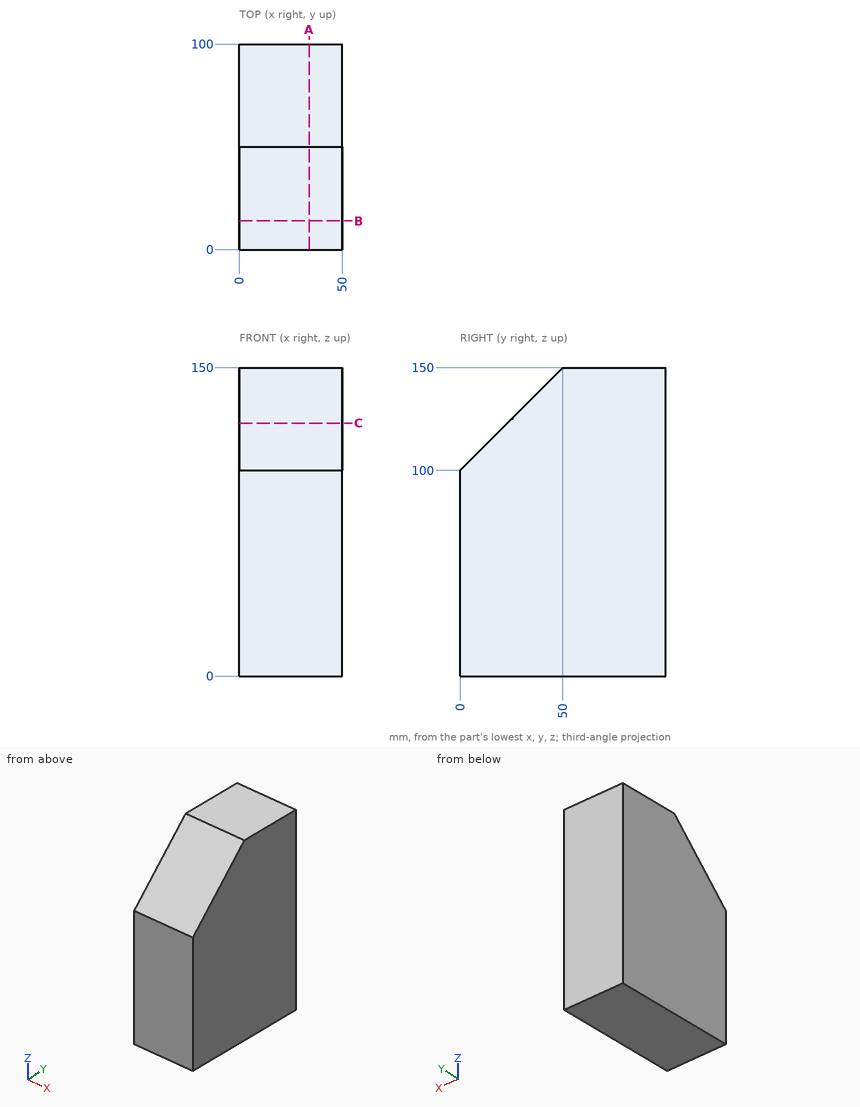
Study the drawing (mm; zero at the part's minimum x, y, z) and answer. Coordinates: 2 decimals unless noted, no trailing zeros. Loops run counter-clockwise (first coordinate to the right, second up) from the corner with the lowest first, then second, coordinate; pieces in that order, holes last. Notation, with made-up numbers: M 80,87.5 L 135,87.5 A29 ccw 135,126.5 Z; hole C -26.75,-15 d10. An arc over 180 degrees is marked long. Answer in a Markdown table with one row per item. Add a question column.
1. Find section A-A, the plane x = 34. Write down the section's boundary in (y, z), then the cut area to 4 significant figures.
2. Flat-ended cylindrical pins translate along their axes: P1, Ø1.5, axis at x = 18.5, y = 19, coming from the +Z side; P2, Ø4, axis at x = 29.5, y = 32.5, coming from the +Z side. Find the tip coordinate at first contact, or state that the pin passes through.
3. Consider L1, parallel to Z at x = 24, y = 17; L2, parallel to Z at x = 18.5, y = 23; L3, parallel to Y at x = 10, z = 133. Determine where each line is inside the solid, lowest interval first.
4. Find section B-B, the plane y = 14. Write down the section's boundary in (x, z).
5. Find section C-C, the plane z = 123. Write down the section's boundary in (x, y), then the cut area to 3 significant figures.
Reported:
| question | item | result |
|---|---|---|
| 1 | outline | M 0,0 L 100,0 L 100,150 L 50,150 L 0,100 Z |
| 1 | area | 13,750 mm^2 |
| 2 | P1 | stops at z = 119.75 |
| 2 | P2 | stops at z = 134.5 |
| 3 | L1 | z = 0 to 117 |
| 3 | L2 | z = 0 to 123 |
| 3 | L3 | y = 33 to 100 |
| 4 | outline | M 0,0 L 50,0 L 50,114 L 0,114 Z |
| 5 | outline | M 0,23 L 50,23 L 50,100 L 0,100 Z |
| 5 | area | 3,850 mm^2 |
